For this review, use the dimensioned drawing (mm, ordinates from the lowest corner) and the shaded views. A direction names the side the tool comes from. Coordinates: 2 decimals unless noted, no trailing zeros. Order: outer loops, then holes, each group sorted by start corner. A loop starts at its lowest first (then second) coordinate and runs counter-clockwise, first axis right, second up. Notation, with made-up numbers: M -30.75,71 L 19.25,71 A26 ccw 19.25,92 Z; hole C 51.25,-22 d11. An arc over 180 degrees is marked long. One line per item, written item: value.
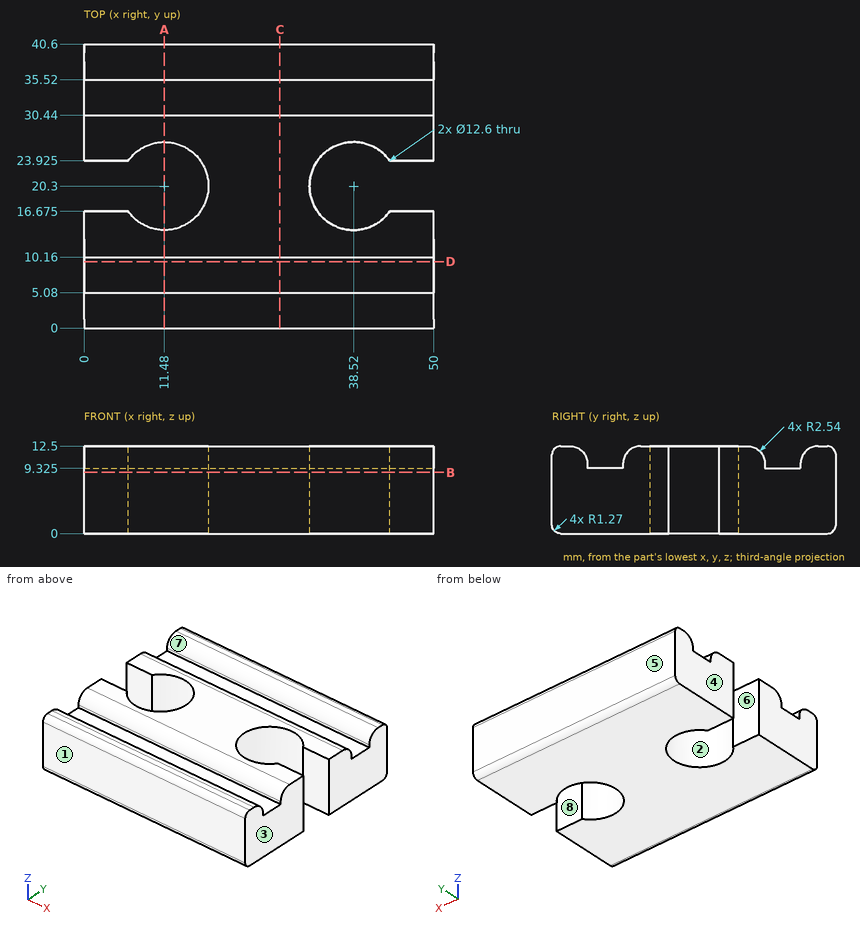
(1) Insertion check: pin 1 Ø4 at (x, z) = (44.5, 7.5) entering from -Y; pin 2 Ø2.5 at (x, y) = (37, 33.5) entering from +Z (3 decimals); pin 3 Ø3 at (y, z) = (20.5, 7) entering from -X. Each pin has a flat end and moves straight along its axis. Give the tip position at first contact, or say it passes through.
Geometry results:
pin 1: stops at y = 0
pin 2: stops at z = 9.325
pin 3: stops at x = 17.55
(2) We need section B-B, the plane z = 8.75. State the section outline as (x, y) points (3 decimals).
Geometry results:
outline: M 0,0 L 50,0 L 50,16.675 L 43.673,16.675 A6.3 cw long 43.673,23.925 L 50,23.925 L 50,40.6 L 0,40.6 L 0,23.925 L 6.327,23.925 A6.3 cw long 6.327,16.675 L 0,16.675 Z
(3) Mouldability with a two-part tool opening along X and no side actions: class the marked faces 1, 2 and 3 as +X half, -X half, draft (parallel to the pull), parting line (faces both ways), or undercut.
Geometry results:
face 1: draft
face 2: undercut
face 3: +X half
(4) We need section C-C, the plane x = 28. State the section outline as (y, z) points (3 decimals).
Geometry results:
outline: M 0,1.27 A1.27 ccw 1.27,0 L 39.33,0 A1.27 ccw 40.6,1.27 L 40.6,11.23 A1.27 ccw 39.33,12.5 L 38.06,12.5 A2.54 ccw 35.52,9.96 L 35.52,9.325 L 30.44,9.325 L 30.44,9.96 A2.54 ccw 27.9,12.5 L 12.7,12.5 A2.54 ccw 10.16,9.96 L 10.16,9.325 L 5.08,9.325 L 5.08,9.96 A2.54 ccw 2.54,12.5 L 1.27,12.5 A1.27 ccw 0,11.23 Z
(5) Tool access review of the marked faces 4, 5, 6, 7 and 8: name each direction out of +Z, -Z, +X, -X, +Y, -Y from which nothing blocks a thin tool from reaching the whole face with its end or side.
Geometry results:
face 4: +Z, -Z, -X, +Y, -Y
face 5: +Z, -Z, +X, -X, +Y
face 6: +Z, -Z, -X
face 7: +Z, +X, -X
face 8: +Z, -Z, +X
(6) We need section A-A, the plane x = 11.48. State the section outline as (y, z) points (3 decimals).
Geometry results:
outline: M 0,1.27 A1.27 ccw 1.27,0 L 14,0 L 14,12.5 L 12.7,12.5 A2.54 ccw 10.16,9.96 L 10.16,9.325 L 5.08,9.325 L 5.08,9.96 A2.54 ccw 2.54,12.5 L 1.27,12.5 A1.27 ccw 0,11.23 Z; M 26.6,0 L 39.33,0 A1.27 ccw 40.6,1.27 L 40.6,11.23 A1.27 ccw 39.33,12.5 L 38.06,12.5 A2.54 ccw 35.52,9.96 L 35.52,9.325 L 30.44,9.325 L 30.44,9.96 A2.54 ccw 27.9,12.5 L 26.6,12.5 Z
(7) We need section D-D, the plane y = 9.5. State the section outline as (x, z) points (3 decimals).
Geometry results:
outline: M 0,0 L 50,0 L 50,9.325 L 0,9.325 Z
(8) For L1, parallel to Y at x = 11.48, z = 9.5; L2, parallel to Y at x = 11.48, z = 6.5; L3, parallel to Y at x = 29.5, z = 11.25, list the stretches that pass through material, from the lowest coordinate up.
Geometry results:
L1: y = 0 to 5.08, 10.16 to 14, 26.6 to 30.44, 35.52 to 40.6
L2: y = 0 to 14, 26.6 to 40.6
L3: y = 0 to 4.73, 10.51 to 30.09, 35.87 to 40.6
